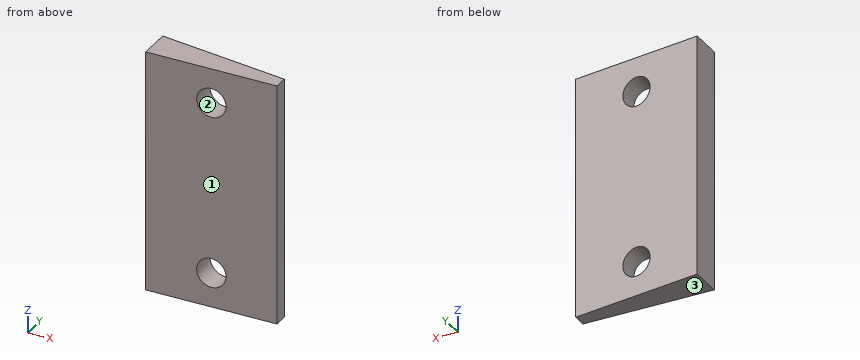
```python
from build123d import *

# Parameters (mm, degrees)
DODANIE_WYCI_GNI_CIE1_DEPTH = 70
SZKIC2_R                    = 4.25
WYTNIJ_WYCI_GNI_CIE1_DEPTH  = 10


with BuildPart() as part:
    # Szkic1 → Dodanie-wyciągnięcie1 (new body)
    with BuildSketch(Plane.XY):
        Polygon((-16.558198873, 5.237130444), (-16.558198873, -4.103421275), (21.441801127, -4.103421275), (21.441801127, -0.103421275), align=None)
    extrude(amount=DODANIE_WYCI_GNI_CIE1_DEPTH)

    # Szkic2 → Wytnij-wyciągnięcie1 (cut)
    with BuildSketch(Plane(origin=(0, 5.237130444, 0), x_dir=(-1, 0, 0), z_dir=(0, -1, 0))):
        with Locations(Location((-2.441801127, -60, 0), (0, 0, 270))):
            Circle(SZKIC2_R)
        with Locations(Location((-2.441801127, -10, 0), (0, 0, 270))):
            Circle(SZKIC2_R)
    extrude(amount=WYTNIJ_WYCI_GNI_CIE1_DEPTH, mode=Mode.SUBTRACT)


solid = part.part
```
For this review, take the finished solid that the model builds, in its own axes (mm). Face numbers are marked on the shaded views. Give positions to 0.01 mm unless a question says otherwise; leave off trailing zeros. Loops run counter-clockwise (first coordinate to the right, second up) from the corner with the lowest first, then second, coordinate; pieces in that order, holes last. Notation, with made-up numbers: M 65.25,6 L 108.25,6 A23 cw 108.25,19 Z; hole C -15,-4 d11. An arc over 180 degrees is marked long. One line per item, written item: value. Start each with the question number.
Q1. Add section D-D (z = 58.5). Give the boundary of the cut face in (x, y), and give its area (3 significant figures).
Q2. Draft analysis for pull direction Z (two halves, no side actions). For the marked faces 1, 2 and 3, state which applies: released by +Z, released by -Z, zero draft, split by the parting line, or undercut.
Q3. Add section C-C (y = 1.25). Give the boundary of the cut face in (x, z).
Q4. Add section B-B (x = 5.5). Give the boundary of the cut face in (y, z), and give its area (3 significant figures).
Q5. Clearance check with a flat-ended pin moving along its axis: pin 1 Ø5 at (x, z) = (1, 39) entering from +Y. State where the tip first meets the part, or that it passes through.
Q6. For L1, parallel to X at y = -2.25, z = 60; L2, parallel to Z at x = 4.5, y = -2.5; L3, parallel to Y at x = 9, z = 15.5, list the stretches that pass through material, from the lowest coordinate up.
Q7. Add section A-A (z = 10). Give the boundary of the cut face in (x, y), and give its area (3 significant figures).
Reply:
1. outline: M -16.56,-4.1 L -1.53,-4.1 L -1.53,3.13 L -16.56,5.24 Z; M 6.42,-4.1 L 21.44,-4.1 L 21.44,-0.1 L 6.42,2.01 Z
1. area: 200 mm²
2. face 1: zero draft
2. face 2: undercut
2. face 3: released by -Z
3. outline: M -16.56,0 L 11.81,0 L 11.81,70 L -16.56,70 Z; hole C 2.44,10 d8.5; hole C 2.44,60 d8.5
4. outline: M -4.1,0 L 2.14,0 L 2.14,7.05 L -4.1,7.05 Z; M -4.1,12.95 L 2.14,12.95 L 2.14,57.05 L -4.1,57.05 Z; M -4.1,62.95 L 2.14,62.95 L 2.14,70 L -4.1,70 Z
4. area: 363 mm²
5. pin 1: y = 3.12
6. L1: -16.56 to -1.81, 6.69 to 21.44
6. L2: 0 to 6.28, 13.72 to 56.28, 63.72 to 70
6. L3: -4.1 to 1.65
7. outline: M -16.56,-4.1 L -1.81,-4.1 L -1.81,3.16 L -16.56,5.24 Z; M 6.69,-4.1 L 21.44,-4.1 L 21.44,-0.1 L 6.69,1.97 Z
7. area: 197 mm²
